Work out the finished part from the listing and answer in its coordinate system (mm). Coordinates: 2 decimals unless noted, no trailing zeros. Loops run counter-clockwise (first coordinate to the right, second up) from the corner with the lowest first, then second, coordinate; pieces in that order, holes last. Notation, with made-up numbers: M -39.75,55 L -23.75,55 A21 ccw -23.75,59 Z; hole C -3,-39 d3. An arc over 180 degrees is marked long. Write each question's results on one line, items separated by ' | '.
```python
from build123d import *

# Parameters (mm, degrees)
SKETCH1_R           = 25
BOSS_EXTRUDE1_DEPTH = 789.6
SKETCH2_R           = 25
SKETCH2_R_2         = 4.7625
CUT_EXTRUDE1_DEPTH  = 74
SKETCH3_R           = 25
SKETCH3_R_2         = 4.7625
CUT_EXTRUDE2_DEPTH  = 100
SKETCH4_R           = 1.5
CUT_EXTRUDE3_DEPTH  = 30
SKETCH5_R           = 4.7625
BOSS_EXTRUDE3_DEPTH = 20
SKETCH6_R           = 4.7625
BOSS_EXTRUDE4_DEPTH = 40


with BuildPart() as part:
    # Sketch1 → Boss-Extrude1 (new body)
    with BuildSketch(Plane(origin=(0, 0, 0), x_dir=(1, 0, 0), z_dir=(0, 1, 0))):
        Circle(SKETCH1_R)
    extrude(amount=BOSS_EXTRUDE1_DEPTH)

    # Sketch2 → Cut-Extrude1 (cut)
    with BuildSketch(Plane(origin=(0, 789.6, 0), x_dir=(1, 0, 0), z_dir=(0, 1, 0))):
        Circle(SKETCH2_R)
        Circle(SKETCH2_R_2, mode=Mode.SUBTRACT)
    extrude(amount=-CUT_EXTRUDE1_DEPTH, mode=Mode.SUBTRACT)

    # Sketch3 → Cut-Extrude2 (cut)
    with BuildSketch(Plane.XZ):
        Circle(SKETCH3_R)
        Circle(SKETCH3_R_2, mode=Mode.SUBTRACT)
    extrude(amount=-CUT_EXTRUDE2_DEPTH, mode=Mode.SUBTRACT)

    # Sketch4 → Cut-Extrude3 (cut)
    with BuildSketch(Plane(origin=(0, 0, 0), x_dir=(0, 0, -1), z_dir=(1, 0, 0))):
        with Locations((3.570652979, 337.95)):
            Circle(SKETCH4_R)
    extrude(amount=-CUT_EXTRUDE3_DEPTH, mode=Mode.SUBTRACT)

    # Sketch5 → Boss-Extrude3 (add)
    with BuildSketch(Plane.XZ):
        Circle(SKETCH5_R)
    extrude(amount=BOSS_EXTRUDE3_DEPTH)

    # Sketch6 → Boss-Extrude4 (add)
    with BuildSketch(Plane(origin=(0, 789.6, 0), x_dir=(1, 0, 0), z_dir=(0, 1, 0))):
        Circle(SKETCH6_R)
    extrude(amount=BOSS_EXTRUDE4_DEPTH)


solid = part.part
```
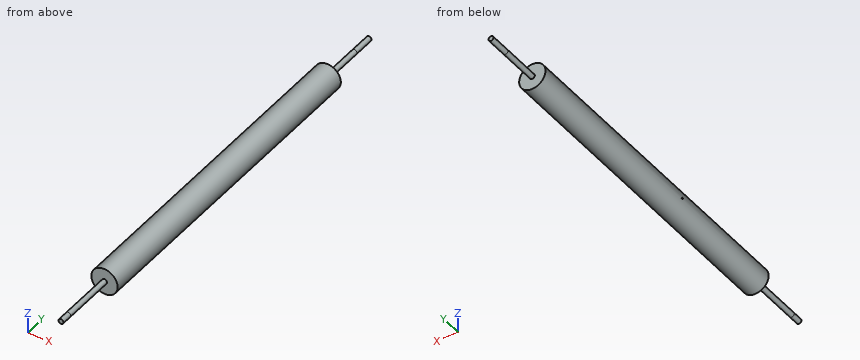
1) Find section A-A, the plane y = 325.5. Give the vertices of the cut face in (x, z), and give its area (3 significant figures).
Check result:
outline: C 0,0 d50 | area: 1,960 mm^2
2) Straight lines are drawn through the part: probe 1 along Y at (x, z) = (-9.5, -7.5); probe 2 along Z at (x, y) = (-13, 337); probe 3 along Z at (x, y) = (-7, 337). For each, find the intervals that lie inside material, in ascending order. Write a range as [from, to].
Check result:
probe 1: [100, 715.6] | probe 2: [-21.35, -4.73], [-2.41, 21.35] | probe 3: [-24, -4.73], [-2.41, 24]
3) Given pin 1 Ø6 at (y, z) = (79, -4.5) entering from -X; pin 2 Ø4 at (y, z) = (555.5, 5.5) entering from +X; pin 3 Ø2 at (x, y) = (-2, 528.5) entering from -Z, each flat-ended and moving along its own axis, determine where each tip first touches the part or whether it passes through.
Check result:
pin 1: x = -4.52 | pin 2: x = 24.75 | pin 3: z = -24.98
4) Find section B-B, the plane x = -13.5. Give the vertices of the cut face in (y, z), and give its area (3 significant figures).
Check result:
outline: M 100,-21.04 L 715.6,-21.04 L 715.6,21.04 L 100,21.04 Z; hole C 337.95,-3.57 d3 | area: 25,900 mm^2
